Read the model definition and answer for the solid it produces. Units are mm, in the model's axes. A direction names the side the tool comes from. Give positions to 0.01 mm unless a question says otherwise; leave off trailing zeros. Use one line per item in the form item = value.
```python
from build123d import *

# Parameters (mm, degrees)
F4_DEPTH = 22.098
F3_W     = 20.574
F3_H     = 48.387
F5_DEPTH = 0.127
F6_DEPTH = 11.557


with BuildPart() as f1:
    # F0 (on Right) → F1 (revolve)
    with BuildSketch(Plane.YZ):
        Polygon((-25.4, 23.4315), (-25.4, 13.9065), (0, 13.9065), (0, 23.5585), align=None)
    revolve(axis=Axis((0, -12.7, 13.9065), (0, 1, 0)))



with BuildPart() as f2:
    # F0 (on Right) → F2 (revolve)
    with BuildSketch(Plane.YZ):
        Polygon((0, -13.9065), (0, -4.2545), (-25.4, -4.2545), (-25.4, -13.7795), align=None)
    revolve(axis=Axis((0, -12.7, -13.843), (0, 0.9999875002, -0.0049999375)))


with BuildPart() as f1_1:
    add(f1.part)

    add(f2.part)  # F4 merges F2
    # F3 (on Front) → F4 (join)
    with BuildSketch(Plane.XZ):
        with BuildLine():
            Line((4.8895, -3.175), (4.8895, 3.175))
            ThreePointArc((4.8895, 3.175), (5.3288232031, 5.3549618496), (6.57820844, 7.1946017797))
            ThreePointArc((6.57820844, 7.1946017797), (0, 4.5085), (-6.57820844, 7.1946017797))
            ThreePointArc((-6.57820844, 7.1946017797), (-5.3288232031, 5.3549618496), (-4.8895, 3.175))
            Line((-4.8895, 3.175), (-4.8895, -3.175))
            ThreePointArc((-4.8895, -3.175), (-5.3287958737, -5.3547810515), (-6.5781006563, -7.1942548506))
            ThreePointArc((-6.5781006563, -7.1942548506), (0, -4.508258706), (6.5781006563, -7.1942548506))
            ThreePointArc((6.5781006563, -7.1942548506), (5.3287958737, -5.3547810515), (4.8895, -3.175))
        make_face()
    extrude(amount=F4_DEPTH)

    # F3 (on Front) → F5 (join, symmetric)
    with BuildSketch(Plane.XZ):
        Rectangle(F3_W, F3_H)
        with BuildLine():
            ThreePointArc((6.57820844, 7.1946017797), (5.3288232031, 5.3549618496), (4.8895, 3.175))
            Line((4.8895, 3.175), (4.8895, -3.175))
            ThreePointArc((4.8895, -3.175), (5.3287958737, -5.3547810515), (6.5781006563, -7.1942548506))
            ThreePointArc((6.5781006563, -7.1942548506), (8.6643924763, -10.2661066466), (9.398, -13.906258706))
            ThreePointArc((9.398, -13.906258706), (-3.6401520595, -22.5706511824), (-6.5781006563, -7.1942548506))
            ThreePointArc((-6.5781006563, -7.1942548506), (-5.3287958737, -5.3547810515), (-4.8895, -3.175))
            Line((-4.8895, -3.175), (-4.8895, 3.175))
            ThreePointArc((-4.8895, 3.175), (-5.3288232031, 5.3549618496), (-6.57820844, 7.1946017797))
            ThreePointArc((-6.57820844, 7.1946017797), (-3.6400824909, 22.5709217037), (9.398, 13.9065))
            ThreePointArc((9.398, 13.9065), (8.6644217037, 10.2664175091), (6.57820844, 7.1946017797))
        make_face(mode=Mode.SUBTRACT)
        with BuildLine():
            ThreePointArc((9.398, -13.906258706), (8.6643924763, -10.2661066466), (6.5781006563, -7.1942548506))
            ThreePointArc((6.5781006563, -7.1942548506), (0, -4.508258706), (-6.5781006563, -7.1942548506))
            ThreePointArc((-6.5781006563, -7.1942548506), (-3.6401520595, -22.5706511824), (9.398, -13.906258706))
        make_face()
        with BuildLine():
            Line((4.8895, -3.175), (4.8895, 3.175))
            ThreePointArc((4.8895, 3.175), (5.3288232031, 5.3549618496), (6.57820844, 7.1946017797))
            ThreePointArc((6.57820844, 7.1946017797), (0, 4.5085), (-6.57820844, 7.1946017797))
            ThreePointArc((-6.57820844, 7.1946017797), (-5.3288232031, 5.3549618496), (-4.8895, 3.175))
            Line((-4.8895, 3.175), (-4.8895, -3.175))
            ThreePointArc((-4.8895, -3.175), (-5.3287958737, -5.3547810515), (-6.5781006563, -7.1942548506))
            ThreePointArc((-6.5781006563, -7.1942548506), (0, -4.508258706), (6.5781006563, -7.1942548506))
            ThreePointArc((6.5781006563, -7.1942548506), (5.3287958737, -5.3547810515), (4.8895, -3.175))
        make_face()
        with BuildLine():
            ThreePointArc((-6.57820844, 7.1946017797), (0, 4.5085), (6.57820844, 7.1946017797))
            ThreePointArc((6.57820844, 7.1946017797), (8.6644217037, 10.2664175091), (9.398, 13.9065))
            ThreePointArc((9.398, 13.9065), (-3.6400824909, 22.5709217037), (-6.57820844, 7.1946017797))
        make_face()
    extrude(amount=F5_DEPTH, both=True)

    # F6 (add): a face of the model
    f6_faces = [f1_1.faces().sort_by_distance(p)[0] for p in [
        (0, 0.127, 0),
    ]]
    extrude(f6_faces, amount=F6_DEPTH)


solid = f1_1.part
```
Item 1: Given pin 1 Ø1.9 at (y, z) = (-14, -0.5) entering from -X; pin 2 Ø3 at (y, z) = (-20.5, -2) entering from +X; pin 3 Ø9.5 at (x, z) = (1.5, -3) entering from -Y, each flat-ended and moving along its own axis, determine where each tip first touches the part or whether it passes through.
Checks:
pin_1 = -4.89
pin_2 = 4.9
pin_3 = -25.41
Item 2: Which of the six approach directions +Z, -Z, +X, -X, +Y, -Y give full straight-line access (tool end or side, diameter ignored) to faces 1 (the cylindrical face through (-5.16, -10.96, 4.9)), 2 (the cylindrical face through (5.12, -10.96, -4.77)), 3 (the conical face through (2.88, -12.94, 23.05)), 4 (the flat face through (0, 6, -24.194))?
Checks:
face_1 = -X, -Y
face_2 = +X, -Y
face_3 = -Y
face_4 = -Z, +X, -X, +Y, -Y
Item 3: Straight lines are drawn through the part: L1, parallel to Y at x = 1, z = -11; L2, parallel to Y at x = 1.5, z = 1.5; L3, parallel to Z at x = 6.75, y = -11.5 (3 decimals). For each, find the intervals that lie inside material, in ascending order. Write a range as from..to.
Checks:
L1 = -25.4..11.68
L2 = -22.1..11.68
L3 = -20.668..-7.03, 7.088..20.725
Item 4: Determine the mould class of faces 5 (the flat face through (-4.89, -11, 0)), 6 (the flat face through (-10.287, 6, 0)), 7 (the flat face through (0, 6, 24.194)) for opening direction Z: +Z half, -Z half, draft (parallel to the pull), parting line (faces both ways), or undercut.
Checks:
face_5 = undercut
face_6 = draft
face_7 = +Z half
